Read the model definition and answer for the solid it produces. Units are mm, in the model's axes. A direction names the side the tool comes from. Give positions to 0.01 mm unless a question says otherwise; leave off trailing zeros. Write each loop counter-clockwise with the first axis right and the second up, starting at its lowest first coordinate (ties: lowest second). Pieces come first, ordered by that corner, then holes. Notation, with made-up numbers: (66, -29.5) - (110, -29.5) arc R26 ccw to (110, -9.5) - close; hole circle Ø2 at (13.25, 51). An arc over 180 degrees is marked (long way). Answer as CSV lines item,"result".
Autodesk Inventor part; units mm, degrees
ref_plane "YZ Plane" through (0, 0, 0) normal (1, 0, 0) x (0, 1, 0)
ref_plane "XZ Plane" through (0, 0, 0) normal (0, 1, 0) x (-1, 0, 0)
ref_plane "XY Plane" through (0, 0, 0) normal (0, 0, 1) x (1, 0, 0)
sketch "Sketch1" plane through (0, 0, 0) normal (0, 0, 1) x (1, 0, 0)
  line L0 (1033.8246, 340.1521) -> (1033.8246, -117.0479)
  line L1 (627.4246, -117.0479) -> (627.4246, 340.1521)
  line L2 (627.4246, -117.0479) -> (1033.8246, -117.0479)
  arc A0 (665.5246, 340.1521) -> (995.7246, 340.1521) centre (830.6246, 678.8187) ccw
  line L3 (627.4246, 340.1521) -> (665.5246, 340.1521)
  line L4 (995.7246, 340.1521) -> (1033.8246, 340.1521)
  point P0 (0, 0)
  dimension "d0" = 406.4
  dimension "d1" = 457.2
extrude "Extrusion1" add sketch "Sketch1" along normal blind 19.05
sketch "Sketch2" plane through (0, 0, 19.05) normal (0, 0, 1) x (1, 0, 0)
  line L0 (1033.8246, 340.1521) -> (627.4246, 340.1521)
  line L1 (627.4246, -117.0479) -> (-960.0754, -117.0479)
  line L2 (627.4246, 340.1521) -> (646.4746, 340.1521)
  line L3 (646.4746, 340.1521) -> (646.4746, -117.0479)
  line L4 (646.4746, -117.0479) -> (627.4246, -117.0479)
  line L5 (627.4246, -117.0479) -> (627.4246, 340.1521)
  line L6 (1033.8246, -117.0479) -> (1033.8246, 340.1521)
  line L7 (1033.8246, 340.1521) -> (1014.7746, 340.1521)
  line L8 (1014.7746, 340.1521) -> (1014.7746, -117.0479)
  line L9 (1014.7746, -117.0479) -> (1033.8246, -117.0479)
  line L10 (1033.8246, -117.0479) -> (1033.8246, 340.1521)
  line L11 (627.4246, 340.1521) -> (627.4246, -117.0479)
  line L12 (627.4246, 263.9521) -> (646.4746, 263.9521)
  line L13 (1014.7746, 263.9521) -> (1033.8246, 263.9521)
  line L14 (627.4246, 187.7521) -> (646.4746, 187.7521)
  line L15 (1014.7746, 187.7521) -> (1033.8246, 187.7521)
  line L16 (627.4246, 111.5521) -> (646.4746, 111.5521)
  line L17 (1014.7746, 111.5521) -> (1033.8246, 111.5521)
  line L18 (627.4246, 35.3521) -> (646.4746, 35.3521)
  line L19 (1014.7746, 35.3521) -> (1033.8246, 35.3521)
  line L20 (1033.8246, -40.8479) -> (1014.7746, -40.8479)
  line L21 (646.4746, -40.8479) -> (627.4246, -40.8479)
  point P0 (0, 0)
  dimension "d7" = 19.05
  dimension "d8" = 19.05
extrude "Extrusion2" cut sketch "Sketch2" against normal blind 19.05 contours L6 L13 L8 L0 | L3 L12 L5 L0 | L6 L17 L8 L15 | L3 L16 L5 L14 | L6 L20 L8 L19 | L3 L21 L5 L18
sketch "Sketch3" plane through (0, 0, 19.05) normal (0, 0, 1) x (1, 0, 0)
  line L0 (1131.5205, 302.0521) -> (511.2286, 302.0521)
  line L1 (1014.7746, 340.1521) -> (995.7246, 340.1521)
  line L2 (1127.4261, 283.0021) -> (305.147, 283.0021)
  line L3 (830.6246, 74.0239) -> (830.6246, 388.6053)
  line L4 (1033.8246, 187.7521) -> (1033.8246, 263.9521)
  line L5 (983.0246, 283.0021) -> (881.4246, 283.0021)
  line L6 (881.4246, 283.0021) -> (881.4246, 263.9521)
  line L7 (881.4246, 263.9521) -> (983.0246, 263.9521)
  line L8 (983.0246, 263.9521) -> (983.0246, 283.0021)
  line L9 (1014.7746, 263.9521) -> (1014.7746, 340.1521)
  line L10 (678.2246, 283.0021) -> (779.8246, 283.0021)
  line L11 (779.8246, 283.0021) -> (779.8246, 263.9521)
  line L12 (779.8246, 263.9521) -> (678.2246, 263.9521)
  line L13 (678.2246, 263.9521) -> (678.2246, 283.0021)
  line L14 (646.4746, 340.1521) -> (646.4746, 263.9521)
  point P0 (0, 0)
  dimension "d24" = 38.1
  dimension "d25" = 19.05
  dimension "d26" = 203.2
  dimension "d27" = 31.75
  dimension "d28" = 101.6
  dimension "d29" = 19.05
  dimension "d30" = 31.75
  dimension "d31" = 101.6
  dimension "d32" = 19.05
extrude "Extrusion3" cut sketch "Sketch3" against normal blind 25.4 contours L8 L7 L6 L2 | L11 L12 L13 L2
sketch "Sketch5" plane through (0, 0, 19.05) normal (0, 0, 1) x (1, 0, 0)
  line L0 (665.5246, 234.6812) -> (995.7246, 234.6812)
  line L1 (995.7246, 234.6812) -> (995.7246, -97.9979)
  line L2 (995.7246, -97.9979) -> (665.5246, -97.9979)
  line L3 (665.5246, -97.9979) -> (665.5246, 234.6812)
  line L4 (1033.8246, 187.7521) -> (1033.8246, 263.9521)
  line L5 (627.4246, -117.0479) -> (1033.8246, -117.0479)
  line L6 (627.4246, 111.5521) -> (627.4246, 35.3521)
  point P0 (0, 0)
  dimension "d35" = 38.1
  dimension "d36" = 19.05
  dimension "d37" = 38.1
extrude "Extrusion4" cut sketch "Sketch5" against normal blind 25.4
properties part number "left side" material "Wood (Birch)"
(1) A cutting plane is placed at D-D (x = 939). Write down the section's boundary in (y, z), and give its area (3 significant figures).
Worked out:
outline,"(-117.05, 0) - (-98, 0) - (-98, 19.05) - (-117.05, 19.05) - close; (234.68, 0) - (263.95, 0) - (263.95, 19.05) - (234.68, 19.05) - close; (283, 0) - (317.98, 0) - (317.98, 19.05) - (283, 19.05) - close"
area,"1,590 mm^2"
(2) A cutting plane is placed at B-B (y = 271.5). Write down the section's boundary in (x, z), and give its area (3 significant figures).
Worked out:
outline,"(646.47, 0) - (678.22, 0) - (678.22, 19.05) - (646.47, 19.05) - close; (779.82, 0) - (881.42, 0) - (881.42, 19.05) - (779.82, 19.05) - close; (983.02, 0) - (1014.77, 0) - (1014.77, 19.05) - (983.02, 19.05) - close"
area,"3,150 mm^2"
(3) A cutting plane is placed at C-C (x = 835.5). Write down the section's boundary in (y, z).
Worked out:
outline,"(-117.05, 0) - (-98, 0) - (-98, 19.05) - (-117.05, 19.05) - close; (234.68, 0) - (302.08, 0) - (302.08, 19.05) - (234.68, 19.05) - close"
(4) A cutting plane is placed at A-A (y = 210). Write down the section's boundary in (x, z).
Worked out:
outline,"(627.42, 0) - (665.52, 0) - (665.52, 19.05) - (627.42, 19.05) - close; (995.72, 0) - (1033.82, 0) - (1033.82, 19.05) - (995.72, 19.05) - close"
(5) For faces 5 (the flat face through (730, 263.952, 10)), 6 (the flat face through (828, -117.048, 9)), 7 (the flat face through (1024, 187.752, 10)), 8 (the flat face through (637, 35.352, 10)), 9 (the flat face through (1033.825, 74, 9)), determine the directions among +Z, -Z, +X, -X, +Y, -Y from which every point of the face is accessible in a straight line to the end or side of a thin tool.
Worked out:
face 5,"+Z, -Z"
face 6,"+Z, -Z, +X, -X, -Y"
face 7,"+Z, -Z, +X"
face 8,"+Z, -Z, -X"
face 9,"+Z, -Z, +X, +Y, -Y"
(6) Each of these flat-tipped pins is pushed along its axis until it touches: P1, Ø5.5, axis at y = -17.5, z = 12, coming from the -X side; P2, Ø9.5, axis at x = 910, z = 13.5, coming from the +Y side; P3, Ø9.5, axis at x = 638, z = 11.5, coming from the +Y side. Where does it stop, or does it pass through?
Worked out:
P1,"stops at x = 646.47"
P2,"stops at y = 311.56"
P3,"stops at y = 263.95"
(7) The mould has two halves that part along X. Classify faces 1 (the flat face through (1014.775, 303, 10)), 2 (the flat face through (665.525, 66, 10)), 3 (the flat face through (646.475, 303, 10)), 4 (the flat face through (656, 340.152, 9)): +X half, -X half, draft (parallel to the pull), parting line (faces both ways), or undercut.
Worked out:
face 1,"+X half"
face 2,"undercut"
face 3,"-X half"
face 4,"draft"
(8) Find the intervals of material crossed by L1, parallel to Y at x = 835, z = 2.25; L2, parallel to X at y = 86.5, z = 3.75; L3, parallel to Y at x = 769.5, z = 2.5, in increasing order.
Worked out:
L1,"y = -117.05 to -98, 234.68 to 302.08"
L2,"x = 627.42 to 665.52, 995.72 to 1033.82"
L3,"y = -117.05 to -98, 234.68 to 263.95, 283 to 307.04"
